Source: CAD feature listing. Evaluate the final solid. Frame: model axes, mm. Give positions to 0.01 mm unless a question says otherwise; leave off trailing zeros. Write each loop counter-clockwise with the first axis right and the second up, starting at its lowest first coordinate (ties: lowest second). Pieces come first, ordered by that corner, then holes. Notation, with made-up numbers: (-33, -16.75) - (6, -16.75) arc R14 cw to (6, -9.75) - close; hole circle Ø9 at (-23.5, 5). An arc over 180 degrees is marked (long way). Answer as a JSON object with one key per item and string values. Group by question number.
from build123d import *

# Parameters (mm, degrees)
SKETCH1_R                         = 53.721
SKETCH1_R_2                       = 50.8
BODY_EXTRUSION_DEPTH              = 457.2
UPPER_BULKHEAD_HOLES_REACH        = 474.717
UPPER_BULKHEAD_HOLES_END_RADIUS   = 50.8
SKETCH2_R                         = 1.7526
UPPER_BULKHEAD_HOLE_PATTERN_COUNT = 4
LOWER_BULKHEAD_HOLES_REACH        = 474.717
LOWER_BULKHEAD_HOLES_END_RADIUS   = 50.8
SKETCH3_R                         = 1.7526
LOWER_BULKHEAD_HOLE_PATTERN_COUNT = 4
SKETCH4_R                         = 3.0226
COUNTERSINK_DEPTH                 = 1.524
COUNTERSINK_PATTERN_COUNT         = 4


with BuildPart() as part:
    # Sketch1 → Body Extrusion (new body)
    with BuildSketch(Plane(origin=(0, 0, 0), x_dir=(1, 0, 0), z_dir=(0, 1, 0))):
        Circle(SKETCH1_R)
        Circle(SKETCH1_R_2, mode=Mode.SUBTRACT)
    extrude(amount=BODY_EXTRUSION_DEPTH)

    # Upper Bulkhead Holes: up to this cylinder (the profile starts outside it)
    upper_bulkhead_holes_end = Plane(origin=(0, 450.85, 0), z_dir=(0, -1, 0)) * Cylinder(UPPER_BULKHEAD_HOLES_END_RADIUS, 1052.034, mode=Mode.PRIVATE)
    # Sketch2 → Upper Bulkhead Holes (cut, up to the surface)
    with BuildSketch(Plane.XY.offset(53.721), mode=Mode.PRIVATE) as upper_bulkhead_holes_sk1:
        with Locations((0, 450.85)):
            Circle(SKETCH2_R)
    upper_bulkhead_holes_tool1 = extrude(upper_bulkhead_holes_sk1.sketch, amount=-UPPER_BULKHEAD_HOLES_REACH, mode=Mode.PRIVATE) - upper_bulkhead_holes_end
    upper_bulkhead_holes = upper_bulkhead_holes_tool1.solids().sort_by_distance((0, 450.85, 53.721))[0]
    add(upper_bulkhead_holes, mode=Mode.SUBTRACT)

    # Upper Bulkhead Hole Pattern: Upper Bulkhead Holes ×4 about axis
    upper_bulkhead_hole_pattern_axis = Axis((0, 457.2, 0), (0, -1, 0))
    for i in range(1, UPPER_BULKHEAD_HOLE_PATTERN_COUNT):
        add(upper_bulkhead_holes.rotate(upper_bulkhead_hole_pattern_axis, i * 360 / UPPER_BULKHEAD_HOLE_PATTERN_COUNT), mode=Mode.SUBTRACT)

    # Lower Bulkhead Holes: up to this cylinder (the profile starts outside it)
    lower_bulkhead_holes_end = Plane(origin=(0, 260.35, 0), z_dir=(0, -1, 0)) * Cylinder(LOWER_BULKHEAD_HOLES_END_RADIUS, 1052.034, mode=Mode.PRIVATE)
    # Sketch3 → Lower Bulkhead Holes (cut, up to the surface)
    with BuildSketch(Plane.XY.offset(53.721), mode=Mode.PRIVATE) as lower_bulkhead_holes_sk1:
        with Locations((0, 260.35)):
            Circle(SKETCH3_R)
    lower_bulkhead_holes_tool1 = extrude(lower_bulkhead_holes_sk1.sketch, amount=-LOWER_BULKHEAD_HOLES_REACH, mode=Mode.PRIVATE) - lower_bulkhead_holes_end
    lower_bulkhead_holes = lower_bulkhead_holes_tool1.solids().sort_by_distance((0, 260.35, 53.721))[0]
    add(lower_bulkhead_holes, mode=Mode.SUBTRACT)

    # Lower Bulkhead Hole Pattern: Lower Bulkhead Holes ×4 about axis
    lower_bulkhead_hole_pattern_axis = Axis((0, 457.2, 0), (0, -1, 0))
    for i in range(1, LOWER_BULKHEAD_HOLE_PATTERN_COUNT):
        add(lower_bulkhead_holes.rotate(lower_bulkhead_hole_pattern_axis, i * 360 / LOWER_BULKHEAD_HOLE_PATTERN_COUNT), mode=Mode.SUBTRACT)

    # Sketch4 → Countersink (cut)
    with BuildSketch(Plane.XY.offset(53.721)):
        with Locations((0, 450.85)):
            Circle(SKETCH4_R)
        with Locations((0, 260.35)):
            Circle(SKETCH4_R)
    countersink = extrude(amount=-COUNTERSINK_DEPTH, mode=Mode.SUBTRACT)

    # Countersink Pattern: Countersink ×4 about axis
    countersink_pattern_axis = Axis((0, 0, 0), (0, 1, 0))
    for i in range(1, COUNTERSINK_PATTERN_COUNT):
        add(countersink.rotate(countersink_pattern_axis, i * 360 / COUNTERSINK_PATTERN_COUNT), mode=Mode.SUBTRACT)


solid = part.part
Q1. First-contact query: pin 1 Ø2 at (x, y) = (-30.5, 142.5) entering from +Z; pin 2 Ø1.8 at (y, z) = (450, -1) entering from +X; pin 3 Ø2 at (y, z) = (104.5, 30) entering from +X. Flat tips, straight axial feed; report the tip coordinate or a pass-through.
Q2. Section B-B on x = -24.5. Return the cut outline in (y, z), then the cut area to 3 significant figures.
Q3. Section C-C on y = 232.5. Return the cut outline in (x, z), then the cut area to 3 significant figures.
Q4. Section A-A on z = -42. Return the cut outline in (x, y), then the cut area to 3 significant figures.
Q5. Ray query, probe 1 along Y at (x, z) = (53, 0); probe 2 along Y at (x, z) = (-51, 0); probe 3 along X at (y, z) = (335.5, -0.5). Return the intervals inside material, ascending. Write a range as [from, to].
Taken from the geometry:
{
 "1": {"pin 1": "stops at z = 44.9", "pin 2": "stops at x = 52.2", "pin 3": "stops at x = 45.22"},
 "2": {"outline": "(0, -47.81) - (457.2, -47.81) - (457.2, -44.5) - (0, -44.5) - close; (0, 44.5) - (457.2, 44.5) - (457.2, 47.81) - (0, 47.81) - close", "area": "3,020 mm²"},
 "3": {"outline": "circle Ø107.44 at (0, 0); hole circle Ø101.6 at (0, 0)", "area": "959 mm²"},
 "4": {"outline": "(-33.5, 0) - (-28.58, 0) - (-28.58, 457.2) - (-33.5, 457.2) - close; (28.58, 0) - (33.5, 0) - (33.5, 457.2) - (28.58, 457.2) - close", "area": "4,500 mm²"},
 "5": {"probe 1": "y = [0, 257.33], [263.37, 447.83], [453.87, 457.2]", "probe 2": "y = [0, 258.6], [262.1, 449.1], [452.6, 457.2]", "probe 3": "x = [-53.72, -50.8], [50.8, 53.72]"}
}
